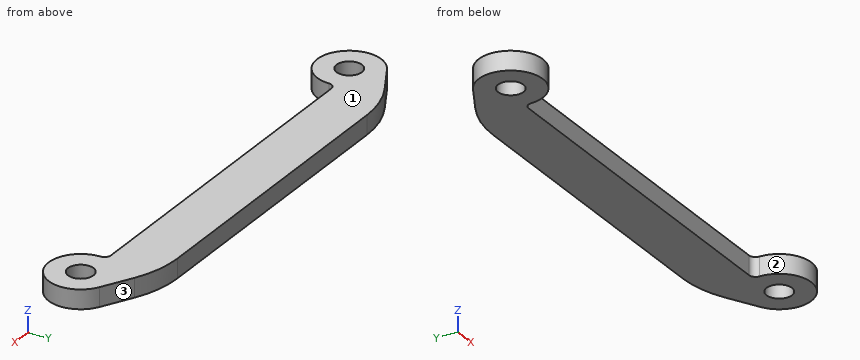
```python
from build123d import *

# Parameters (mm, degrees)
SKETCH1_R           = 1.5875
BOSS_EXTRUDE1_DEPTH = 1.190625
FILLET1_R           = 12.7
FILLET1_2_R         = 0.8128


with BuildPart() as part:
    # Sketch1 → Boss-Extrude1 (new body, symmetric)
    with BuildSketch(Plane.XY):
        with BuildLine():
            Line((-22.225, 0), (22.225, 0))
            Line((22.225, 0), (28.841565542, -3.6137254))
            ThreePointArc((28.841565542, -3.6137254), (28.965173596, -10.565282887), (22.9235, -7.1247))
            Line((22.9235, -7.1247), (22.9235, -6.35))
            Line((22.9235, -6.35), (-22.9235, -6.35))
            Line((-22.9235, -6.35), (-22.9235, -7.1247))
            ThreePointArc((-22.9235, -7.1247), (-28.965173596, -10.565282887), (-28.841565542, -3.6137254))
            Line((-28.841565542, -3.6137254), (-22.225, 0))
        make_face()
        with Locations((-26.924, -7.1247)):
            Circle(SKETCH1_R, mode=Mode.SUBTRACT)
        with Locations((26.924, -7.1247)):
            Circle(SKETCH1_R, mode=Mode.SUBTRACT)
    extrude(amount=BOSS_EXTRUDE1_DEPTH, both=True)

    # Fillet1
    fillet1_edges = [part.edges().sort_by_distance(p)[0] for p in [
        (-22.225, 0, 0),
        (22.225, 0, 0),
    ]]
    fillet(fillet1_edges, radius=FILLET1_R)

    # Fillet1 2
    fillet1_2_edges = [part.edges().sort_by_distance(p)[0] for p in [
        (-22.9235, -6.35, 0),
        (22.9235, -6.35, 0),
    ]]
    fillet(fillet1_2_edges, radius=FILLET1_2_R)


solid = part.part
```
Could you check a few things on this model? Use its own coordinates, in mm. Face numbers are marked on the shaded views. Give positions to 0.01 mm unless a question says otherwise; leave off trailing zeros. Write each loop counter-clockwise with the first axis right and the second up, starting at its lowest first coordinate (ties: lowest second). Pieces come first, ordered by that corner, then holes. Notation, with made-up numbers: (85, 86) - (101, 86) arc R37 cw to (101, 122) - close; hole circle Ø2 at (31, 28). An arc over 180 degrees is marked (long way). One line per item, written item: value. Start each with the question number.
Item 1: Please list where these lines run through material, in increasing order: line 1 (X direction, y = -6, z = 0.8); line 2 (Y direction, x = -5, z = 0.7); line 3 (X direction, y = -8.75, z = 0.4). Write a range as from..to.
Item 2: Imagine slicing it at B-B, the plane z = 0.1. Give the number of separate pieces and of enclosed holes in the cut face, and give its area (3 significant figures).
Item 3: I'm going to push flat-ended pins straight in: pin 1 (1 mm diameter, centred on x = 1, y = -8, fed in from -Z); pin 2 (1 mm diameter, centred on y = -8.5, z = -0.5, fed in from -X). Where does each tip first touch, or does it pass through?
Item 4: Imagine slicing it at A-A, the plane y = -9.5. List the corners of the cut face in (x, z) for me (3 decimals).
Item 5: If we mould it in two halves opening along X, with no side actions, what happens to the marked faces 1, 2 and 3? For each: +X half, -X half, draft (parallel to the pull), parting line (faces both ways), or undercut.
Item 6: Imagine slicing it at C-C, the plane x = 11.5. List the corners of the cut face in (y, z) for me.
Item 7: Imagine slicing it at D-D, the plane y = -1. List the corners of the cut face in (x, z) for me.
Geometry says:
1. line 1: -30.76..-28.04, -25.8..25.8, 28.04..30.76
1. line 2: -6.35..0
1. line 3: -30.58..-23.27, 23.27..30.58
2. separate pieces: 1
2. enclosed holes: 2
2. area: 395 mm^2
3. pin 1: through
3. pin 2: x = -30.83
4. outline: (-30.143, -1.191) - (-23.705, -1.191) - (-23.705, 1.191) - (-30.143, 1.191) - close; (23.705, -1.191) - (30.143, -1.191) - (30.143, 1.191) - (23.705, 1.191) - close
5. face 1: draft
5. face 2: undercut
5. face 3: +X half
6. outline: (-6.35, -1.19) - (0, -1.19) - (0, 1.19) - (-6.35, 1.19) - close
7. outline: (-23.92, -1.19) - (23.92, -1.19) - (23.92, 1.19) - (-23.92, 1.19) - close
